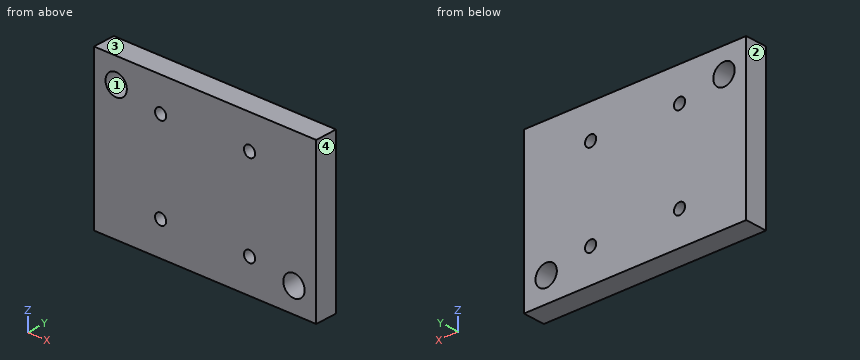
from build123d import *

# Parameters (mm, degrees)
ESQUISSE1_W                               = 50
ESQUISSE1_H                               = 35
BOSS_EXTRU_1_DEPTH                        = 5
TROU_POUR_TARAUDAGE_POUR_TROU_TARAUD_M3_D = 2.5
D_GAGEMENT_M43_D                          = 4.8


with BuildPart() as part:
    # Esquisse1 → Boss.-Extru.1 (new body)
    with BuildSketch(Plane(origin=(0, 0, 0), x_dir=(1, 0, 0), z_dir=(0, 1, 0))):
        with Locations((6.571428571, -2.357142857)):
            Rectangle(ESQUISSE1_W, ESQUISSE1_H)
    extrude(amount=BOSS_EXTRU_1_DEPTH)

    # Trou pour taraudage pour trou taraudé M33 (through all)
    with Locations(Plane(origin=(0, 5, 0), x_dir=(1, 0, 0), z_dir=(0, 1, 0))):
        with Locations((16.571428571, 7.642857143), (-3.428571429, 7.642857143), (16.571428571, -12.357142857), (-3.428571429, -12.357142857)):
            Hole(TROU_POUR_TARAUDAGE_POUR_TROU_TARAUD_M3_D / 2)

    # Dégagement M43 (through all)
    with Locations(Plane(origin=(0, 5, 0), x_dir=(1, 0, 0), z_dir=(0, 1, 0))):
        with Locations((26.571428571, 9.642857143), (-13.428571429, -14.357142857)):
            Hole(D_GAGEMENT_M43_D / 2)


solid = part.part
Here's how the part is built. I have some questions about the finished solid (model axes, mm). Face numbers are marked on the shaded views. Round coordinates to 2 decimals unless told otherwise and drop trailing zeros. Write each loop counter-clockwise with the first axis right and the second up, starting at its lowest first coordinate (ties: lowest second). Pieces come first, ordered by that corner, then holes. Notation, with made-up numbers: (12.5, 13.25) -> (53.5, 13.25) arc R21 ccw to (53.5, 48.25) -> close; hole circle Ø9 at (18, -37.75). An arc over 180 degrees is marked (long way). One line per item, written item: value.
1) We'd pull the mould along X, two halves only. Please class the marked faces 1, 2, 3 and 4: released by +X, released by -X, zero draft, split by the parting line, or undercut.
Filled sheet:
face 1: undercut
face 2: released by -X
face 3: zero draft
face 4: released by +X
2) Suppose I cut it at B-B on y = 2.5. List the corners of the cut face in (x, z) for me.
Filled sheet:
outline: (-18.43, -15.14) -> (31.57, -15.14) -> (31.57, 19.86) -> (-18.43, 19.86) -> close; hole circle Ø4.8 at (-13.43, 14.36); hole circle Ø2.5 at (-3.43, -7.64); hole circle Ø2.5 at (-3.43, 12.36); hole circle Ø2.5 at (16.57, -7.64); hole circle Ø2.5 at (16.57, 12.36); hole circle Ø4.8 at (26.57, -9.64)
3) If I drill on line 1 (X direction, y = 2.7, z = 11.5); line 2 (X direction, y = 3.85, z = -11.5); line 3 (Z direction, x = 25, y = 1.5), over which ranges is the centre line in solid material (lowest first)? Write a range as [from, to].
Filled sheet:
line 1: x = [-18.43, -4.34], [-2.52, 15.66], [17.48, 31.57]
line 2: x = [-18.43, 25.05], [28.09, 31.57]
line 3: z = [-15.14, -11.46], [-7.83, 19.86]
4) Suppose I cut it at A-A on x = 16. List the corners of the cut face in (y, z) for me.
Filled sheet:
outline: (0, -15.14) -> (5, -15.14) -> (5, -8.75) -> (0, -8.75) -> close; (0, -6.53) -> (5, -6.53) -> (5, 11.25) -> (0, 11.25) -> close; (0, 13.47) -> (5, 13.47) -> (5, 19.86) -> (0, 19.86) -> close
5) Suppose I cut it at C-C on x = -14.5. List the corners of the cut face in (y, z) for me.
Filled sheet:
outline: (0, -15.14) -> (5, -15.14) -> (5, 12.21) -> (0, 12.21) -> close; (0, 16.5) -> (5, 16.5) -> (5, 19.86) -> (0, 19.86) -> close
